Can you work these out from the model? Positions are in its coordinate system, mm. Face numbers are marked on the shaded views. A direction names the side the tool comes from. Round coordinates to 2 decimals unless told otherwise and drop trailing zeros. Loops run counter-clockwise (first coordinate to the right, second up) from the corner with the lowest first, then second, coordinate; pieces in that order, holes last. Notation, with made-up numbers: (57.5, 78.25) -> (100.5, 78.25) arc R24 ccw to (100.5, 103.25) -> close; hole circle Ø9 at (35.25, 71.25). An arc over 180 degrees is marked (long way). Use a Markdown table: item, result.
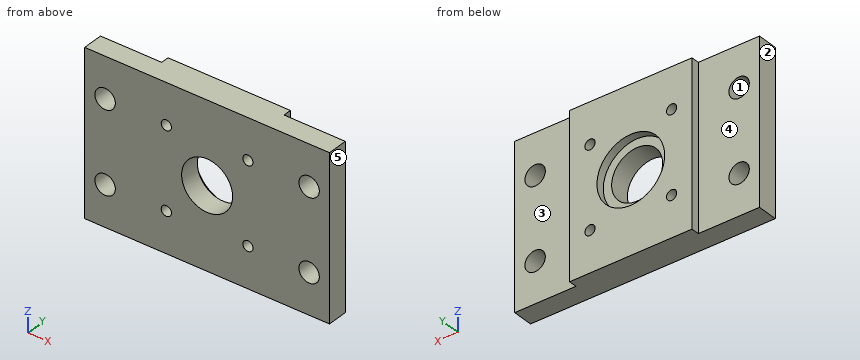
from build123d import *

# Parameters (mm, degrees)
SKETCH1_W            = 60
SKETCH1_H            = 40
SKETCH1_R            = 2.5
SKETCH1_R_2          = 6.25
BODY_DEPTH           = 5
SKETCH3_W            = 30
SKETCH3_H            = 40
SKETCH3_R            = 8.3
BEARING_PLACE_DEPTH  = 2
SKETCH4_R            = 1.25
FIXATION_HOLES_DEPTH = 37.728735344


with BuildPart() as part:
    # Sketch1 → Body (new body)
    with BuildSketch(Plane(origin=(0, 0, 0), x_dir=(1, 0, 0), z_dir=(0, 1, 0))):
        Rectangle(SKETCH1_W, SKETCH1_H)
        with Locations(Location((25, 10, 0), (0, 0, 270))):
            Circle(SKETCH1_R, mode=Mode.SUBTRACT)
        with Locations(Location((25, -10, 0), (0, 0, 270))):
            Circle(SKETCH1_R, mode=Mode.SUBTRACT)
        with Locations(Location((0, 0, 0), (0, 0, 270))):
            Circle(SKETCH1_R_2, mode=Mode.SUBTRACT)
        with Locations(Location((-25, -10, 0), (0, 0, 90))):
            Circle(SKETCH1_R, mode=Mode.SUBTRACT)
        with Locations(Location((-25, 10, 0), (0, 0, 90))):
            Circle(SKETCH1_R, mode=Mode.SUBTRACT)
    extrude(amount=BODY_DEPTH)

    # Sketch3 → Bearing_Place (add)
    with BuildSketch(Plane(origin=(0, 5, 0), x_dir=(1, 0, 0), z_dir=(0, 1, 0))):
        Rectangle(SKETCH3_W, SKETCH3_H)
        with Locations(Location((0, 0, 0), (0, 0, 270))):
            Circle(SKETCH3_R, mode=Mode.SUBTRACT)
    extrude(amount=BEARING_PLACE_DEPTH)

    # Sketch4 → Fixation_Holes (cut, through all)
    with BuildSketch(Plane(origin=(0, 7, 0), x_dir=(1, 0, 0), z_dir=(0, 1, 0))):
        with Locations(Location((-10, 10, 0), (0, 0, 270))):
            Circle(SKETCH4_R)
        with Locations(Location((10, 10, 0), (0, 0, 270))):
            Circle(SKETCH4_R)
        with Locations(Location((10, -10, 0), (0, 0, 270))):
            Circle(SKETCH4_R)
        with Locations(Location((-10, -10, 0), (0, 0, 270))):
            Circle(SKETCH4_R)
    extrude(amount=-FIXATION_HOLES_DEPTH, mode=Mode.SUBTRACT)


solid = part.part
1. I want a section at D-D (x = 0). Please give me the cut outline in (y, z).
Answer sheet:
| item | result |
|---|---|
| outline | (0, -20) -> (7, -20) -> (7, -8.3) -> (5, -8.3) -> (5, -6.25) -> (0, -6.25) -> close; (0, 6.25) -> (5, 6.25) -> (5, 8.3) -> (7, 8.3) -> (7, 20) -> (0, 20) -> close |
2. I need wall thicknesses on line 1 (Z direction, x = -25, y = 2.75); line 2 (X direction, y = 2.75, z = 10); line 3 (Y direction, x = -19, z = 8). Which ranges of each line are inside material? Lowest first, please.
Answer sheet:
| item | result |
|---|---|
| line 1 | z = -20 to -12.5, -7.5 to 7.5, 12.5 to 20 |
| line 2 | x = -30 to -27.5, -22.5 to -11.25, -8.75 to 8.75, 11.25 to 22.5, 27.5 to 30 |
| line 3 | y = 0 to 5 |
3. I want a section at B-B (x = -10). Please give me the cut outline in (y, z).
Answer sheet:
| item | result |
|---|---|
| outline | (0, -20) -> (7, -20) -> (7, -11.25) -> (0, -11.25) -> close; (0, -8.75) -> (7, -8.75) -> (7, 8.75) -> (0, 8.75) -> close; (0, 11.25) -> (7, 11.25) -> (7, 20) -> (0, 20) -> close |
4. If we mould it in two halves opening along X, with no side actions, what happens to the marked faces 1, 2 and 3? For each: +X half, -X half, draft (parallel to the pull), parting line (faces both ways), or undercut.
Answer sheet:
| item | result |
|---|---|
| face 1 | undercut |
| face 2 | -X half |
| face 3 | draft |
5. I want a section at A-A (z = 0). Please give me the cut outline in (x, y).
Answer sheet:
| item | result |
|---|---|
| outline | (-30, 0) -> (-6.25, 0) -> (-6.25, 5) -> (-8.3, 5) -> (-8.3, 7) -> (-15, 7) -> (-15, 5) -> (-30, 5) -> close; (6.25, 0) -> (30, 0) -> (30, 5) -> (15, 5) -> (15, 7) -> (8.3, 7) -> (8.3, 5) -> (6.25, 5) -> close |
6. I want a section at C-C (y = 3.5). State how many separate pieces and enclosed holes the cut face has, plus the area to 3 significant figures.
Answer sheet:
| item | result |
|---|---|
| separate pieces | 1 |
| enclosed holes | 9 |
| area | 2,180 mm² |
7. Will these pins go through, and if not, where does the flat tip stop? pin 1 Ø10 at (x, z) = (0, 0) entering from -Y; pin 2 Ø0.6 at (y, z) = (6, 8) entering from -X; pin 3 Ø6 at (x, z) = (-25, -10) entering from +Y.
Answer sheet:
| item | result |
|---|---|
| pin 1 | passes through |
| pin 2 | stops at x = -15 |
| pin 3 | stops at y = 5 |
8. Which directions (+Z, -Z, +X, -X, +Y, -Y) give clear straight access to the entire face, cutting with the end or side of a thin tool? Please do the marked faces 4 and 5.
Answer sheet:
| item | result |
|---|---|
| face 4 | +Z, -Z, -X, +Y |
| face 5 | +Z, -Z, +X, +Y, -Y |
